Read the model definition and answer for the solid it produces. Units are mm, in the model's axes. Coordinates: 2 decimals unless noted, no trailing zeros. Loops run counter-clockwise (first coordinate to the right, second up) from the corner with the lowest first, then second, coordinate; pieces in that order, holes last.
Q1. Straight lines are drawn through the part: line 1 (Z direction, x = 164, y = 2.2); line 2 (Z direction, x = 140, y = 1.5); line 3 (Z direction, x = 82, y = 2.6). For each, find the intervals that lie inside material, in ascending order.
Q2. Section A-A (y = 1.55) is taken. Count the separate pieces of the cut face and the enclosed holes in it, then the cut area to 3 significant figures.
Q3. Section B-B (x = 80.5) is taken. Give the vertices of the cut face in (y, z) (3 decimals).
Q4. The mould has two halves that part along X. Classify faces 1 (the face through (130, 3.175, -9)), 2 (the face through (130.226, 1.565, -20.613)): pulls with the +X half, pulls with the -X half, needs draft (parallel to the pull), parting line crosses it, or undercut.
Q5. Flat-ended cylindrical pins translate along their axes: P1, Ø1, axis at x = 56, y = 2.5, coming from the -Z side; P2, Ø1.8, axis at x = 116, z = -3.13, coming from the -Y side; P3, Ø1.6, axis at y = 1, z = -20.5, coming from the -X side. Find the tip coordinate at first contact, or state that the pin passes through.
from build123d import *

# Parameters (mm, degrees)
SKETCH1_W           = 264
SKETCH1_H           = 27.40559892
SKETCH1_R           = 2
SKETCH1_R_2         = 1.5
BOSS_EXTRUDE1_DEPTH = 3.175
SKETCH2_R           = 1.5
CUT_EXTRUDE1_DEPTH  = 10
SKETCH3_W           = 90
SKETCH3_H           = 10
CUT_EXTRUDE2_DEPTH  = 10
CUT_EXTRUDE3_START  = -10
SKETCH4_R           = 2
CUT_EXTRUDE3_DEPTH  = 10


with BuildPart() as part:
    # Sketch1 → Boss-Extrude1 (new body)
    with BuildSketch(Plane(origin=(0, 0, 0), x_dir=(1, 0, 0), z_dir=(0, 1, 0))):
        with Locations((132, 11.832834683)):
            Rectangle(SKETCH1_W, SKETCH1_H)
        with Locations(Location((132, 21.535634143, 0), (0, 0, 270))):
            Circle(SKETCH1_R, mode=Mode.SUBTRACT)
        with Locations(Location((68, 21.535634143, 0), (0, 0, 270))):
            Circle(SKETCH1_R, mode=Mode.SUBTRACT)
        with Locations(Location((196, 21.535634143, 0), (0, 0, 270))):
            Circle(SKETCH1_R, mode=Mode.SUBTRACT)
        with Locations(Location((260, 3.130035223, 0), (0, 0, 270))):
            Circle(SKETCH1_R_2, mode=Mode.SUBTRACT)
        with Locations(Location((4, 3.130035223, 0), (0, 0, 270))):
            Circle(SKETCH1_R_2, mode=Mode.SUBTRACT)
        with Locations(Location((36, 3.130035223, 0), (0, 0, 270))):
            Circle(SKETCH1_R_2, mode=Mode.SUBTRACT)
        with Locations(Location((228, 3.130035223, 0), (0, 0, 270))):
            Circle(SKETCH1_R_2, mode=Mode.SUBTRACT)
        with Locations(Location((164, 21.535634143, 0), (0, 0, 270))):
            Circle(SKETCH1_R, mode=Mode.SUBTRACT)
        with Locations(Location((100, 21.535634143, 0), (0, 0, 270))):
            Circle(SKETCH1_R, mode=Mode.SUBTRACT)
    extrude(amount=BOSS_EXTRUDE1_DEPTH)

    # Sketch2 → Cut-Extrude1 (cut)
    with BuildSketch(Plane(origin=(0, 3.175, 0), x_dir=(1, 0, 0), z_dir=(0, 1, 0))):
        with Locations(Location((116, 3.130035223, 0), (0, 0, 270))):
            Circle(SKETCH2_R)
        with Locations(Location((148, 3.130035223, 0), (0, 0, 270))):
            Circle(SKETCH2_R)
        with Locations(Location((100, 3.130035223, 0), (0, 0, 270))):
            Circle(SKETCH2_R)
        with Locations(Location((164, 3.130035223, 0), (0, 0, 270))):
            Circle(SKETCH2_R)
    extrude(amount=-CUT_EXTRUDE1_DEPTH, mode=Mode.SUBTRACT)

    # Sketch3 → Cut-Extrude2 (cut)
    with BuildSketch(Plane(origin=(0, 3.175, 0), x_dir=(1, 0, 0), z_dir=(0, 1, 0))):
        with Locations((45, 20.535634143)):
            Rectangle(SKETCH3_W, SKETCH3_H)
        with Locations((219, 20.535634143)):
            Rectangle(SKETCH3_W, SKETCH3_H)
    extrude(amount=-CUT_EXTRUDE2_DEPTH, mode=Mode.SUBTRACT)

    # Sketch4 → Cut-Extrude3 (cut)
    with BuildSketch(Plane(origin=(0, 3.175, 0), x_dir=(1, 0, 0), z_dir=(0, 1, 0)).offset(CUT_EXTRUDE3_START)):
        with Locations(Location((100, 21.535634143, 0), (0, 0, 270))):
            Circle(SKETCH4_R)
        with Locations(Location((108, 21.535634143, 0), (0, 0, 270))):
            Circle(SKETCH4_R)
        with Locations(Location((116, 21.535634143, 0), (0, 0, 270))):
            Circle(SKETCH4_R)
        with Locations(Location((124, 21.535634143, 0), (0, 0, 270))):
            Circle(SKETCH4_R)
        with Locations(Location((132, 21.535634143, 0), (0, 0, 270))):
            Circle(SKETCH4_R)
        with Locations(Location((140, 21.535634143, 0), (0, 0, 270))):
            Circle(SKETCH4_R)
        with Locations(Location((148, 21.535634143, 0), (0, 0, 270))):
            Circle(SKETCH4_R)
        with Locations(Location((156, 21.535634143, 0), (0, 0, 270))):
            Circle(SKETCH4_R)
        with Locations(Location((164, 21.535634143, 0), (0, 0, 270))):
            Circle(SKETCH4_R)
    extrude(amount=CUT_EXTRUDE3_DEPTH, mode=Mode.SUBTRACT)


solid = part.part
Numbers:
1. line 1: z = -25.54 to -23.54, -19.54 to -4.63, -1.63 to 1.87
1. line 2: z = -25.54 to -23.54, -19.54 to 1.87
1. line 3: z = -15.54 to 1.87
2. separate pieces: 1
2. enclosed holes: 17
2. area: 5,270 mm2
3. outline: (0, -15.536) - (3.175, -15.536) - (3.175, 1.87) - (0, 1.87) - close
4. face 1: needs draft
4. face 2: undercut
5. P1: stops at z = -15.54
5. P2: passes through
5. P3: stops at x = 90
